Autodesk Inventor part; units mm, degrees
ref_plane "YZ Plane" through (0, 0, 0) normal (1, 0, 0) x (0, 1, 0)
ref_plane "XZ Plane" through (0, 0, 0) normal (0, 1, 0) x (-1, 0, 0)
ref_plane "XY Plane" through (0, 0, 0) normal (0, 0, 1) x (1, 0, 0)
sketch "TFT LCD Touch Screen" plane through (0, 0, 0) normal (0, 0, 1) x (1, 0, 0)
  line L0 (-40, 29) -> (40, 29)
  line L1 (40, 29) -> (40, -29)
  line L2 (40, -29) -> (-40, -29)
  line L3 (-40, -29) -> (-40, 29)
  line L4 (-55, 32.5) -> (55, 32.5)
  line L5 (55, 32.5) -> (55, -32.5)
  line L6 (55, -32.5) -> (-55, -32.5)
  line L7 (-55, -32.5) -> (-55, 32.5)
  circle A0 centre (-51, 28.5) radius 1.5
  circle A1 centre (-51, -28.5) radius 1.5
  circle A2 centre (51, -28.5) radius 1.5
  circle A3 centre (51, 28.5) radius 1.5
  point P0 (0.75, 3.075)
  point P1 (0, 29)
  point P2 (-40, 0)
  point P3 (0, 32.5)
  point P4 (55, 0)
  dimension "d0" = 110
  dimension "d1" = 65
  dimension "d2" = 3
  dimension "d3" = 57
  dimension "d4" = 102
  dimension "d5" = 4
  dimension "d6" = 4
  dimension "d7" = 80
  dimension "d8" = 58
sketch "Sketch1" plane through (0, 0, 0) normal (0, 0, 1) x (1, 0, 0)
  line L0 (-40, 29) -> (40, 29)
  line L1 (40, 29) -> (40, -29)
  line L2 (40, -29) -> (-40, -29)
  line L3 (-40, -29) -> (-40, 29)
  line L4 (-55, 32.5) -> (55, 32.5)
  line L5 (55, 32.5) -> (55, -32.5)
  line L6 (55, -32.5) -> (-55, -32.5)
  line L7 (-55, -32.5) -> (-55, 32.5)
  circle A0 centre (-51, 28.5) radius 1.5
  circle A1 centre (-51, -28.5) radius 1.5
  circle A2 centre (51, -28.5) radius 1.5
  circle A3 centre (51, 28.5) radius 1.5
  point P0 (0, 0)
  point P1 (-55, 0)
extrude "Extrusion1" add sketch "Sketch1" against normal blind 1.5 contours L0 L1 L2 L3 | L4 L5 L6 L7
extrude "Extrusion2" add sketch "Sketch1" along normal blind 5 contours L0 L1 L2 L3
sketch "Sketch2" plane through (0, 0, 5) normal (0, 0, 1) x (1, 0, 0)
  line L0 (-40, 29) -> (40, 29)
  line L1 (40, 29) -> (40, -29)
  line L2 (40, -29) -> (-40, -29)
  line L3 (-40, -29) -> (-40, 29)
  line L4 (35.6625, 24.6625) -> (-35.6625, 24.6625)
  line L5 (-35.6625, 24.6625) -> (-35.6625, -24.6625)
  line L6 (-35.6625, -24.6625) -> (35.6625, -24.6625)
  line L7 (35.6625, -24.6625) -> (35.6625, 24.6625)
  point P0 (0, 0)
extrude "Extrusion3" cut sketch "Sketch2" against normal blind 0.2 contours L7 L6 L5 L4
fillet "Fillet1" radius 2 4 edges at (55, 32.5, -0.75) (-55, 32.5, -0.75) (-55, -32.5, -0.75) (55, -32.5, -0.75)
equation "\"d5\" = -0.5 * d3 + 0.5 * d1"
equation "\"d6\" = -0.5 * d4 + 0.5 * d0"
properties part number "TFT Screen"
Geometry: final body of the model. Coordinates: model frame, mm. A direction names the side the tool comes from. Coordinates: 2 decimals unless noted, no trailing zeros. Write each loop counter-clockwise with the first axis right and the second up, starting at its lowest first coordinate (ties: lowest second). Pieces come first, ordered by that corner, then holes. Notation, with made-up numbers: M 1,31 L 12,31 A20 cw 12,46 Z; hole C -24.5,-17 d5. An arc over 180 degrees is marked long. Answer as CSV lines item,"result". Start each with the question number.
Q1. Line query: line 1 (Y direction, x = -51, z = -1); line 2 (Y direction, x = -27.5, z = 3); line 3 (X direction, y = 27, z = 4). Output: solid intervals per line, ascending. Write a range as from..to.
Q2. Cut plane A-A on x = 51. Return the cut outline in (y, z), then the cut area to 3 significant figures.
Q3. Mould query, pull axis X, two halves, no side actions, for faces 5 (the flat face through (40, 0, 2)), 6 (the cylindrical face through (-52.11, 29.51, -0.74)), 7 (the cylindrical face through (49.89, -27.49, -0.74)), 8 (the flat face through (-1, 29, 2)). Classes: released by +X, released by -X, zero draft, split by the parting line, or undercut.
Q4. Cut plane D-D on z = 3.5. Return the cut outline in (x, y).
Q5. Cut plane C-C on x = 0. Return the cut outline in (y, z).
Q6. Pin query (flat end, axial travel): P1, Ø3, axis at x = -3, z = 2.5, coming from the -Y side; P2, Ø1.5, axis at x = -3.5, y = -19.5, coming from the +Z side; P3, Ø1, axis at y = -25, z = 2, coming from the -X side; P4, Ø2.5, axis at x = 51, y = 28.5, coming from the +Z side. Return the tip coordinate at first contact, or that it passes through.
Q7. Cut plane B-B on y = 9. Return the cut outline in (x, z), then the cut area to 3 significant figures.
Q8. Reachability of faces 1 (the flat face through (-40, 0, 2)), 2 (the flat face through (-1, 0, -1.5)), 3 (the flat face through (1, -29, 2)), 4 (the flat face through (0, 0, 4.8)) from +Z, -Z, +X, -X, +Y, -Y: full face, straight path, thin tool, end or side. Return the list, or none.
Findings below:
1,line 1,"y = -32.5..-30, -27..27, 30..32.5"
1,line 2,"y = -29..29"
1,line 3,"x = -40..40"
2,outline,"M -32.5,-1.5 L -30,-1.5 L -30,0 L -32.5,0 Z; M -27,-1.5 L 27,-1.5 L 27,0 L -27,0 Z; M 30,-1.5 L 32.5,-1.5 L 32.5,0 L 30,0 Z"
2,area,"88.5 mm2"
3,face 5,"released by +X"
3,face 6,"undercut"
3,face 7,"undercut"
3,face 8,"zero draft"
4,outline,"M -40,-29 L 40,-29 L 40,29 L -40,29 Z"
5,outline,"M -32.5,-1.5 L 32.5,-1.5 L 32.5,0 L 29,0 L 29,5 L 24.66,5 L 24.66,4.8 L -24.66,4.8 L -24.66,5 L -29,5 L -29,0 L -32.5,0 Z"
6,P1,"stops at y = -29"
6,P2,"stops at z = 4.8"
6,P3,"stops at x = -40"
6,P4,"passes through"
7,outline,"M -55,-1.5 L 55,-1.5 L 55,0 L 40,0 L 40,5 L 35.66,5 L 35.66,4.8 L -35.66,4.8 L -35.66,5 L -40,5 L -40,0 L -55,0 Z"
7,area,"551 mm2"
8,face 1,"+Z, -X, +Y, -Y"
8,face 2,"-Z, +X, -X, +Y, -Y"
8,face 3,"+Z, +X, -X, -Y"
8,face 4,"+Z"
